Verification items for the finished model (mm, model axes). Face numbers are marked on the shaded views. A direction names the side the tool comes from. Round coordinates to 2 decimals unless told otherwise and drop trailing zeros. Write each loop counter-clockwise with the first axis right and the second up, starting at its lowest first coordinate (ties: lowest second). Pieces come first, ordered by that corner, then holes. Notation, with made-up numbers: (20.25, -15.5) -> (32.25, -15.5) arc R31 cw to (32.25, 11.5) -> close; hole circle Ø7 at (-5.5, 38). An arc over 180 degrees is marked (long way). Answer as a JSON object with one key per item and string values. Group by question number.
(1) Gauge pin test, flat ends, axial feed: pin 1 Ø12 at (x, y) = (-9, -63.5) entering from -Z; pin 2 Ø5 at (x, z) = (-2, 3) entering from -Y; pin 3 Ø1.1 at (x, z) = (-17.5, 0) entering from +Y; pin 4 Ø1.5 at (y, z) = (-56.5, 0) entering from -X. Record the tip position at first contact, or that the pin passes through.
(2) Sectioned sample at A-A on z = -1.25. Record the cut outline in (x, y).
(3) Set-up check for the marked faces 1, 2 and 3: record each of +Z, -Z, +X, -X, +Y, -Y from which the full face is reachable in a straight line by a thin tool's end or side.
(4) Scan lines: L1, parallel to X at y = -38, z = -5.75; L2, parallel to Y at x = 22, z = -3.25; L3, parallel to X at y = -10.5, z = -7. Record each from-to range of solid material in increasing order. Write a range as from..to.
(5) Sectioned sample at B-B on x = 12. Record the cut outline in (y, z), and give its area (3 significant figures).
(6) Sectioned sample at C-C on y = -35.5. Record the cut outline in (x, z).
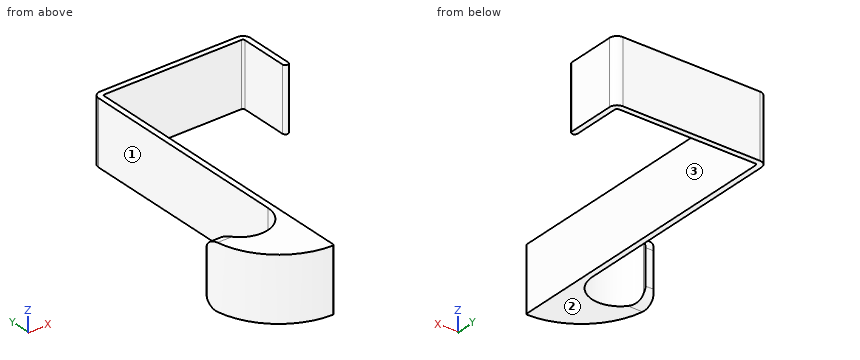
```python
from build123d import *

# Parameters (mm, degrees)
F1_DEPTH = 9
F3_START = -10
F3_DEPTH = 20


with BuildPart() as f1:
    # F0 (on Top) → F1 (new body, symmetric)
    with BuildSketch(Plane.XY):
        with BuildLine():
            ThreePointArc((41.6, -15.8), (42.4, -16.6), (43.2, -15.8))
            Line((43.2, -15.8), (43.2, -2.1))
            ThreePointArc((43.2, -2.1), (42.5849242405, -0.6150757595), (41.1, 0))
            Line((41.1, 0), (2.1, 0))
            ThreePointArc((2.1, 0), (0.6150757595, -0.6150757595), (0, -2.1))
            Line((0, -2.1), (0, -63.6))
            ThreePointArc((0, -63.6), (-7.1872847082, -71.5586113019), (-15.8348734636, -65.2170212766))
            ThreePointArc((-15.8348734636, -65.2170212766), (-17.3482014958, -64.1072430222), (-18.6059763198, -65.5))
            ThreePointArc((-18.6059763198, -65.5), (-12.8679094974, -79.60535621), (1.0873134933, -85.6994710718))
            ThreePointArc((1.0873134933, -85.6994710718), (1.4490392146, -85.5576426968), (1.6, -85.1996320452))
            Line((1.6, -85.1996320452), (1.6, -2.1))
            ThreePointArc((1.6, -2.1), (1.7464466094, -1.7464466094), (2.1, -1.6))
            Line((2.1, -1.6), (41.1, -1.6))
            ThreePointArc((41.1, -1.6), (41.4535533906, -1.7464466094), (41.6, -2.1))
            Line((41.6, -2.1), (41.6, -15.8))
        make_face()
    extrude(amount=F1_DEPTH, both=True)

    # F2 (on Right) → F3 (cut)
    with BuildSketch(Plane.YZ.offset(F3_START)):
        with BuildLine():
            ThreePointArc((-64.7, -5), (-65.8715728753, -7.8284271247), (-68.7, -9))
            Line((-68.7, -9), (-68.7, -10))
            Line((-68.7, -10), (-63.7, -10))
            Line((-63.7, -10), (-63.7, 10))
            Line((-63.7, 10), (-68.7, 10))
            Line((-68.7, 10), (-68.7, 9))
            ThreePointArc((-68.7, 9), (-65.8715728753, 7.8284271247), (-64.7, 5))
            Line((-64.7, 5), (-64.7, -5))
        make_face()
    extrude(amount=-F3_DEPTH, mode=Mode.SUBTRACT)


solid = f1.part
```
Computed values:
{
 "1": {"pin 1": "through", "pin 2": "y = -85.68", "pin 3": "y = -64.7", "pin 4": "x = 0"},
 "2": {"outline": "(-18.61, -65.5) arc R20.21 ccw to (1.09, -85.7) arc R0.5 ccw to (1.6, -85.2) -> (1.6, -2.1) arc R0.5 cw to (2.1, -1.6) -> (41.1, -1.6) arc R0.5 cw to (41.6, -2.1) -> (41.6, -15.8) arc R0.8 ccw to (43.2, -15.8) -> (43.2, -2.1) arc R2.1 ccw to (41.1, 0) -> (2.1, 0) arc R2.1 ccw to (0, -2.1) -> (0, -63.6) arc R8 cw to (-15.83, -65.22) arc R1.4 ccw to (-16.06, -64.7) -> (-18.35, -64.7) arc R1.4 ccw to start"},
 "3": {"face 1": "+Z, -Z, -X, +Y", "face 2": "-Z, +X, -X, +Y, -Y", "face 3": "+Z, -Z, -Y"},
 "4": {"L1": "0..1.6", "L2": "-1.6..0", "L3": "0..1.6, 41.6..43.2"},
 "5": {"outline": "(-1.6, -9) -> (0, -9) -> (0, 9) -> (-1.6, 9) -> close", "area": "28.8 mm2"},
 "6": {"outline": "(0, -9) -> (1.6, -9) -> (1.6, 9) -> (0, 9) -> close"}
}
